from build123d import *

# Parameters (mm, degrees)
SKETCH1_R               = 4.7625
BOSS_EXTRUDE1_DEPTH     = 38.1
SKETCH2_R               = 2.0066
CUT_EXTRUDE1_DEPTH      = 10.414
SKETCH3_R               = 1.1303
CUT_EXTRUDE2_DEPTH      = 8.6868
SKETCH4_R               = 5.084796601
SKETCH4_R_2             = 3.175
CUT_EXTRUDE3_DEPTH      = 9.525
CUT_EXTRUDE4_DEPTH      = 39.690733028
CUT_EXTRUDE4_DEPTH_BACK = 39.690733028
SKETCH5_R               = 0.7874
SKETCH6_R               = 3.5000057
CUT_EXTRUDE5_DEPTH      = 2.50000008
CUT_EXTRUDE7_START      = -0.7366
SKETCH7_R               = 4.7625
SKETCH7_R_2             = 2.667
CUT_EXTRUDE7_DEPTH      = 0.7366


with BuildPart() as part:
    # Sketch1 → Boss-Extrude1 (new body)
    with BuildSketch(Plane(origin=(0, 0, 0), x_dir=(0, 0, -1), z_dir=(1, 0, 0))):
        with Locations(Location((0, 0, 0), (0, 0, 180))):
            Circle(SKETCH1_R)
    extrude(amount=BOSS_EXTRUDE1_DEPTH)

    # Sketch2 → Cut-Extrude1 (cut)
    with BuildSketch(Plane(origin=(38.1, 0, 0), x_dir=(0, 0, -1), z_dir=(1, 0, 0))):
        Circle(SKETCH2_R)
    extrude(amount=-CUT_EXTRUDE1_DEPTH, mode=Mode.SUBTRACT)

    # Sketch3 → Cut-Extrude2 (cut)
    with BuildSketch(Plane(origin=(0, 0, 0), x_dir=(1, 0, 0), z_dir=(0, 1, 0))):
        with Locations(Location((30.48, 0, 0), (0, 0, 90))):
            Circle(SKETCH3_R)
    extrude(amount=CUT_EXTRUDE2_DEPTH, mode=Mode.SUBTRACT)

    # Sketch4 → Cut-Extrude3 (cut)
    with BuildSketch(Plane.ZY):
        Circle(SKETCH4_R)
        Circle(SKETCH4_R_2, mode=Mode.SUBTRACT)
    extrude(amount=-CUT_EXTRUDE3_DEPTH, mode=Mode.SUBTRACT)

    # Sketch5 → Cut-Extrude4 (cut, two sides: drawn at the far end of the back side and taken through both)
    with BuildSketch(Plane(origin=(0, 0, 0), x_dir=(1, 0, 0), z_dir=(0, 1, 0)).offset(-CUT_EXTRUDE4_DEPTH_BACK)):
        with Locations(Location((6.35, 0, 0), (0, 0, 270))):
            Circle(SKETCH5_R)
    extrude(amount=CUT_EXTRUDE4_DEPTH + CUT_EXTRUDE4_DEPTH_BACK, mode=Mode.SUBTRACT)

    # Sketch6 → Cut-Extrude5 (cut)
    with BuildSketch(Plane(origin=(38.1, 0, 0), x_dir=(0, 0, -1), z_dir=(1, 0, 0))):
        Circle(SKETCH6_R)
    extrude(amount=-CUT_EXTRUDE5_DEPTH, mode=Mode.SUBTRACT)

    # Sketch7 → Cut-Extrude7 (cut)
    with BuildSketch(Plane(origin=(35.56, 0, 0), x_dir=(0, 0, -1), z_dir=(1, 0, 0)).offset(CUT_EXTRUDE7_START)):
        with Locations(Location((0, 0, 0), (0, 0, 180))):
            Circle(SKETCH7_R)
        Circle(SKETCH7_R_2, mode=Mode.SUBTRACT)
    extrude(amount=CUT_EXTRUDE7_DEPTH, mode=Mode.SUBTRACT)


solid = part.part
For this review, take the finished solid that the model builds, in its own axes (mm). A direction names the side the tool comes from. Round coordinates to 2 decimals unless told otherwise and drop trailing zeros. Order: outer loops, then holes, each group sorted by start corner. A loop starts at its lowest first (then second) coordinate and runs counter-clockwise, first axis right, second up. Notation, with made-up numbers: M 89.5,73.25 L 104.5,73.25 A29 ccw 104.5,106.25 Z; hole C 36.25,35.25 d11. An arc over 180 degrees is marked long. Write each question's results on one line, items separated by ' | '. Start each with the question number.
1. Tool access review of faces 1 (the face through (36.867, 0.154, 3.497)), 2 (the face through (22, -4.72, -0.62)), 3 (the face through (34.823, 2, 2)), 4 (the face through (4.7, -3.1, -0.69)): name each direction out of +Z, -Z, +X, -X, +Y, -Y from which nothing blocks a thin tool from reaching the whole face with its end or side.
2. To check wall thickness, follow L1, parallel to X at y = 1.5, z = 0; L2, parallel to X at y = -4, z = 2.5 (3 decimals); L3, parallel to Y at x = 37.3, z = 0. State the ranges of each line that lie inside material, in increasing order. Write a range as [from, to].
3. Add section A-A (z = 0). State how many separate pieces and enclosed holes the cut face has, then the cut area to 3 significant figures.
4. Add section C-C (x = 8). State the section outline as (y, z) points (3 decimals).
5. Clearance check with flat-ended pins moving along their axes: pin 1 Ø1.5 at (x, y) = (15.5, -3) entering from -Z; pin 2 Ø3 at (x, y) = (22.5, 2.5) entering from +Z; pin 3 Ø1.2 at (y, z) = (0.5, -0.5) entering from +X. State where each tip first meets the part, or that it passes through.
6. Draft analysis for pull direction X (two halves, no side actions). For faces 5 (the face through (38.1, -4, 0)), 6 (the face through (31.583, 3.191, 0.245)), 7 (the face through (36.81, 4.65, -1.03)), state which applies: pulls with the +X half, pulls with the -X half, needs draft (parallel to the pull), parting line crosses it, or undercut.
7. Add section D-D (x = 34). State the section outline as (y, z) points (1 decimal), then the cut area to 3 significant figures.
Output values:
1) face 1: +X | face 2: +X, -X | face 3: none | face 4: -X
2) L1: [0, 5.56], [7.14, 27.69] | L2: [9.525, 34.823], [35.56, 38.1] | L3: [-4.76, -3.5], [3.5, 4.76]
3) separate pieces: 3 | enclosed holes: 0 | area: 264 mm^2
4) outline: C 0,0 d6.35
5) pin 1: z = -4.2 | pin 2: z = 4.66 | pin 3: x = 27.69
6) face 5: pulls with the +X half | face 6: undercut | face 7: needs draft
7) outline: C 0,0 d9.5; hole C 0,0 d4 | area: 58.6 mm^2
